Autodesk Inventor part; units mm, degrees
ref_plane "YZ Plane" through (0, 0, 0) normal (1, 0, 0) x (0, 1, 0)
ref_plane "XZ Plane" through (0, 0, 0) normal (0, 1, 0) x (-1, 0, 0)
ref_plane "XY Plane" through (0, 0, 0) normal (0, 0, 1) x (1, 0, 0)
sketch "Sketch1" plane through (0, 0, 0) normal (0, 1, 0) x (-1, 0, 0)
  line L0 (0, 108) -> (0, 0)
  line L1 (0, 0) -> (10.412, 0)
  line L2 (10.412, 0) -> (80.1677, 18.691)
  line L3 (80.1677, 18.691) -> (80.1677, 89.309)
  line L4 (80.1677, 89.309) -> (10.412, 108)
  line L5 (10.412, 108) -> (0, 108)
  line L6 (2.5529, 107) -> (1, 101.2044) construction
  line L7 (1, 101.2044) -> (68.6148, 83.0871) construction
  line L8 (68.6148, 83.0871) -> (70.1677, 88.8827) construction
  line L9 (70.1677, 88.8827) -> (2.5529, 107) construction
  line L10 (1, 6.7956) -> (2.5529, 1) construction
  line L11 (2.5529, 1) -> (70.1677, 19.1173) construction
  line L12 (70.1677, 19.1173) -> (68.6148, 24.9129) construction
  line L13 (68.6148, 24.9129) -> (1, 6.7956) construction
  line L14 (71.1677, 88.309) -> (77.1677, 88.309) construction
  line L15 (77.1677, 88.309) -> (77.1677, 19.691) construction
  line L16 (77.1677, 19.691) -> (71.1677, 19.691) construction
  line L17 (71.1677, 19.691) -> (71.1677, 88.309) construction
  line L18 (17.0418, 103.1177) -> (15.4889, 97.3222)
  line L19 (15.4889, 97.3222) -> (23.2163, 95.2516)
  line L20 (23.2163, 95.2516) -> (24.7692, 101.0472)
  line L21 (24.7692, 101.0472) -> (17.0418, 103.1177)
  line L22 (47.9514, 94.8355) -> (46.3985, 89.0399)
  line L23 (46.3985, 89.0399) -> (54.1259, 86.9694)
  line L24 (54.1259, 86.9694) -> (55.6788, 92.765)
  line L25 (55.6788, 92.765) -> (47.9514, 94.8355)
  line L26 (15.4889, 10.6778) -> (17.0418, 4.8823)
  line L27 (17.0418, 4.8823) -> (24.7692, 6.9528)
  line L28 (24.7692, 6.9528) -> (23.2163, 12.7484)
  line L29 (23.2163, 12.7484) -> (15.4889, 10.6778)
  line L30 (46.3985, 18.9601) -> (47.9514, 13.1645)
  line L31 (47.9514, 13.1645) -> (55.6788, 15.235)
  line L32 (55.6788, 15.235) -> (54.1259, 21.0306)
  line L33 (54.1259, 21.0306) -> (46.3985, 18.9601)
  line L34 (54.9024, 89.8672) -> (69.3913, 85.9849) construction
  line L35 (16.2653, 7.7801) -> (1.7765, 3.8978) construction
  line L36 (54.9024, 18.1328) -> (69.3913, 22.0151) construction
  line L37 (16.2653, 100.2199) -> (1.7765, 104.1022) construction
  line L38 (71.1677, 80.309) -> (77.1677, 80.309)
  line L39 (77.1677, 80.309) -> (77.1677, 72.309)
  line L40 (77.1677, 72.309) -> (71.1677, 72.309)
  line L41 (71.1677, 72.309) -> (71.1677, 80.309)
  line L42 (71.1677, 35.691) -> (77.1677, 35.691)
  line L43 (77.1677, 35.691) -> (77.1677, 27.691)
  line L44 (77.1677, 27.691) -> (71.1677, 27.691)
  line L45 (71.1677, 27.691) -> (71.1677, 35.691)
  line L46 (74.1677, 80.309) -> (74.1677, 88.309) construction
  line L47 (74.1677, 27.691) -> (74.1677, 19.691) construction
  dimension "d0" = 70
  dimension "d1" = 6
  dimension "d3" = 70
  dimension "d4" = 6
  dimension "d7" = 3
  dimension "d8" = 3
  dimension "d9" = 6
  dimension "d10" = 3
  dimension "d11" = 1
  dimension "d12" = 1
  dimension "d13" = 1
  dimension "d14" = 1
  dimension "d15" = 15
  dimension "d16" = 1
  dimension "d17" = 1
  dimension "d18" = 1
  dimension "d19" = 108
  dimension "d20" = 8
  dimension "d21" = 15
  dimension "d22" = 8
extrude "Extrusion7" add sketch "Sketch1" along normal blind 6
sketch "Sketch7" plane through (0, 0, 0) normal (0, -1, 0) x (1, 0, 0)
  line L0 (0, 0) -> (0, 108)
  line L1 (0, 92) -> (-6, 92)
  line L2 (-6, 92) -> (-6, 76)
  line L3 (-6, 76) -> (0, 76)
  line L4 (0, 76) -> (0, 92)
  dimension "d74" = 16
  dimension "d75" = 16
  dimension "d76" = 6
extrude "Extrusion8" cut sketch "Sketch7" against normal blind 6
sketch "Sketch8" plane through (0, 0, 0) normal (0, -1, 0) x (1, 0, 0)
  line L0 (-77.1677, 72.309) -> (-71.1677, 35.691) construction
  line L1 (-77.1677, 35.691) -> (-71.1677, 72.309) construction
  circle A0 centre (-74.1677, 54) radius 2.25
  dimension "d80" = 4.5
extrude "Extrusion9" cut sketch "Sketch8" against normal blind 6
sketch "Sketch9" plane through (0, 0, 0) normal (0, -1, 0) x (1, 0, 0)
  line L0 (-46.3985, 18.9601) -> (-24.7692, 6.9528) construction
  line L1 (-23.2163, 12.7484) -> (-47.9514, 13.1645) construction
  circle A0 centre (-35.5839, 12.9564) radius 2.25
  dimension "d83" = 4.5
extrude "Extrusion10" cut sketch "Sketch9" against normal blind 6
sketch "Sketch10" plane through (0, 0, 0) normal (0, -1, 0) x (1, 0, 0)
  line L0 (0, 0) -> (0, 76)
  line L1 (0, 68.25) -> (0, 63.75)
  line L2 (-16.3, 63.75) -> (-16.3, 68.25)
  line L3 (-12.3, 70.75) -> (-5, 70.75)
  line L4 (-5, 61.25) -> (-12.3, 61.25)
  line L5 (-16.3, 68.25) -> (-12.3, 68.25)
  line L6 (-5, 68.25) -> (0, 68.25)
  line L7 (0, 63.75) -> (-5, 63.75)
  line L8 (-12.3, 63.75) -> (-16.3, 63.75)
  line L9 (-12.3, 61.25) -> (-12.3, 63.75)
  line L10 (-12.3, 68.25) -> (-12.3, 70.75)
  line L11 (-5, 70.75) -> (-5, 68.25)
  line L12 (-5, 63.75) -> (-5, 61.25)
  line L13 (0, 34.25) -> (0, 29.75)
  line L14 (-16.3, 29.75) -> (-16.3, 34.25)
  line L15 (-12.3, 36.75) -> (-5, 36.75)
  line L16 (-5, 27.25) -> (-12.3, 27.25)
  line L17 (-16.3, 34.25) -> (-12.3, 34.25)
  line L18 (-5, 34.25) -> (0, 34.25)
  line L19 (0, 29.75) -> (-5, 29.75)
  line L20 (-12.3, 29.75) -> (-16.3, 29.75)
  line L21 (-12.3, 27.25) -> (-12.3, 29.75)
  line L22 (-12.3, 34.25) -> (-12.3, 36.75)
  line L23 (-5, 36.75) -> (-5, 34.25)
  line L24 (-5, 29.75) -> (-5, 27.25)
  point P0 (0, 108)
  point P1 (-16.3, 66)
  point P2 (-16.3, 32)
  dimension "d86" = 4.5
  dimension "d87" = 2.5
  dimension "d88" = 2.5
  dimension "d89" = 5
  dimension "d90" = 7.3
  dimension "d91" = 4
  dimension "d92" = 4.5
  dimension "d93" = 2.5
  dimension "d94" = 2.5
  dimension "d95" = 5
  dimension "d96" = 7.3
  dimension "d97" = 4
  dimension "d98" = 42
  dimension "d99" = 34
extrude "Extrusion11" cut sketch "Sketch10" against normal blind 6
sketch "Sketch11" plane through (0, 0, 0) normal (0, -1, 0) x (1, 0, 0)
  line L0 (0, 68.25) -> (0, 76)
  line L1 (0, 108) -> (-10.412, 108)
  line L2 (-23.2163, 95.2516) -> (-24.7692, 101.0472)
  line L3 (-46.4441, 73.7575) -> (-22.296, 80.228) construction
  line L4 (-22.296, 80.228) -> (-21.9078, 78.7791) construction
  line L5 (-21.9078, 78.7791) -> (-46.0559, 72.3086) construction
  line L6 (-46.0559, 72.3086) -> (-46.4441, 73.7575) construction
  line L7 (-47.0565, 74.1111) -> (-21.9424, 80.8404)
  line L8 (-21.9424, 80.8404) -> (-21.2954, 78.4256)
  line L9 (-21.2954, 78.4256) -> (-46.4095, 71.6963)
  line L10 (-46.4095, 71.6963) -> (-47.0565, 74.1111)
  dimension "d102" = 25
  dimension "d103" = 1.5
  dimension "d104" = 0.5
  dimension "d105" = 22.296
  dimension "d106" = 27.772
extrude "Extrusion12" cut sketch "Sketch11" against normal blind 6
chamfer "Chamfer2" distance 2 angle 45 2 edges at (-80.1677, 3, 89.309) (-80.1677, 3, 18.691)
sketch "Sketch12" plane through (0, 0, 0) normal (0, -1, 0) x (1, 0, 0)
  line L0 (0, 0) -> (0, 29.75)
  line L1 (0, 34.25) -> (0, 63.75)
  line L2 (0, 92) -> (0, 108)
  line L3 (0, 108) -> (-10.412, 108)
  line L4 (0, 102) -> (4, 102)
  line L5 (6, 100) -> (6, 96)
  line L6 (4, 94) -> (0, 94)
  line L7 (0, 94) -> (0, 102)
  line L8 (0, 58) -> (4, 58)
  line L9 (6, 56) -> (6, 52)
  line L10 (4, 50) -> (0, 50)
  line L11 (0, 50) -> (0, 58)
  line L12 (0, 14) -> (4, 14)
  line L13 (6, 12) -> (6, 8)
  line L14 (4, 6) -> (0, 6)
  line L15 (0, 6) -> (0, 14)
  arc A0 (6, 100) -> (4, 102) centre (4, 100) ccw
  arc A1 (4, 94) -> (6, 96) centre (4, 96) ccw
  arc A2 (6, 56) -> (4, 58) centre (4, 56) ccw
  arc A3 (4, 50) -> (6, 52) centre (4, 52) ccw
  arc A4 (4, 6) -> (6, 8) centre (4, 8) ccw
  arc A5 (6, 12) -> (4, 14) centre (4, 12) ccw
  dimension "d112" = 2
  dimension "d113" = 8
  dimension "d114" = 8
  dimension "d115" = 8
  dimension "d116" = 6
  dimension "d117" = 6
  dimension "d118" = 36
  dimension "d119" = 36
extrude "Extrusion13" add sketch "Sketch12" against normal blind 6
equation "\"d3\" = d0"
equation "\"d4\" = d1"
equation "\"d8\" = d7"
equation "\"d9\" = d1"
equation "\"d10\" = d7"
equation "\"d12\" = d11"
equation "\"d88\" = d87"
equation "\"d94\" = d93"
properties part number "front_panel_2004_brace_left"
Here's how the part is built. I have some questions about the finished solid (model axes, mm). A direction names the side the tool comes from. Coordinates: 2 decimals unless noted, no trailing zeros. Order: outer loops, then holes, each group sorted by start corner. A loop starts at its lowest first (then second) coordinate and runs counter-clockwise, first axis right, second up. Notation, with made-up numbers: M 6,9.25 L 15,9.25 A7 ccw 15,21.25 Z; hole C 19,-11 d6. An arc over 180 degrees is marked long. Answer as CSV lines item,"result". Start each with the question number.
1. I want a section at A-A, the plane x = -3.5. Write out the boundary of the cut face in (y, z), and give its area (3 significant figures).
2. For pin 1 (3 mm diameter, centred on y = 4.5, z = 48, fed in from +X); pin 2 (1.2 mm diameter, centred on x = 2, y = 3.5, fed in from +Z); pin 3 (2.5 mm diameter, centred on x = -35.58, z = 12.96, fed in from +Y); pin 4 (3 mm diameter, centred on x = -74, y = 3, fed in from +Z), each with a flat end and sliding along its axis, tell me the tip position at first contact or that it passes through.
3. I want a section at C-C, the plane x = -40. Write out the boundary of the cut face in (y, z), and give its area (3 significant figures).
4. On a 3-axis mill with a long thin cutter (end or side, diameter ignored), from which of +Z, -Z, +X, -X, +Y, -Y can I reach the whole of each face in a straight line? I mean faces 5 (the flat face through (-79.188, 2.958, 19.415)), 6 (the flat face through (-46.73, 2.96, 72.89)), 7 (the flat face through (0, 3, 42)). Say none if no direction works.
5. I need wall thicknesses on line 1 (Z direction, x = -11, y = 4.15); line 2 (Z direction, x = -35.5, y = 0.35); line 3 (X direction, y = 4.15, z = 31). Which ranges of each line are inside material? Lowest first, please. Write a range as [from, to].
6. We'd pull the mould along Z, two halves only. Please class faces 1 (the flat face through (-5, 3, 0)), 2 (the flat face through (-36, 6, 55)), 3 (the flat face through (0, 3, 61)), 4 (the flat face through (-54.913, 2.958, 18.092)): released by +Z, released by -Z, zero draft, split by the parting line, or undercut.
7. I want a section at D-D, the plane y = 4.9. Count the separate pieces of the cut face and the enclosed holes in it, and give its area (3 significant figures).
8. I want a section at B-B, the plane z = 54. Write out the boundary of the cut face in (x, y), and give its area (3 significant figures).
Recorded:
1,outline,"M 0,0 L 6,0 L 6,29.75 L 0,29.75 Z; M 0,34.25 L 6,34.25 L 6,63.75 L 0,63.75 Z; M 0,68.25 L 6,68.25 L 6,76 L 0,76 Z; M 0,92 L 6,92 L 6,108 L 0,108 Z"
1,area,"498 mm2"
2,pin 1,"stops at x = 0"
2,pin 2,"stops at z = 102"
2,pin 3,"passes through"
2,pin 4,"stops at z = 91.36"
3,outline,"M 0,7.93 L 6,7.93 L 6,73.41 L 0,73.41 Z; M 0,76 L 6,76 L 6,100.07 L 0,100.07 Z"
3,area,"537 mm2"
4,face 5,"-Z, -X, +Y, -Y"
4,face 6,"+Y, -Y"
4,face 7,"+X, +Y, -Y"
5,line 1,"z = [0.16, 27.25], [36.75, 61.25], [70.75, 107.84]"
5,line 2,"z = [6.72, 10.71], [15.2, 74.62], [77.21, 101.28]"
5,line 3,"x = [-80.17, -77.17], [-71.17, -16.3]"
6,face 1,"released by -Z"
6,face 2,"zero draft"
6,face 3,"undercut"
6,face 4,"undercut"
7,separate pieces,"1"
7,enclosed holes,"9"
7,area,"6,790 mm2"
8,outline,"M -80.17,0 L -76.42,0 L -76.42,6 L -80.17,6 Z; M -71.92,0 L 6,0 L 6,6 L -71.92,6 Z"
8,area,"490 mm2"
